The figure shows three views and two pictorial views of one solid part (mm, origin at its lowest corner). Answer the questions. Give positions to 0.01 mm unless a question says otherwise; leave off trailing zeros. Write each loop counter-clockwise with the first axis right and the second up, starting at its lowest first coordinate (ties: lowest second). Pieces come first, ordered by that corner, then holes. Notation, with made-up numbers: M 3.25,70.5 L 61.25,70.5 A15 cw 61.25,82.5 Z; hole C 34,81 d2. An arc over 180 degrees is marked long. Return JSON: item names as keys, results as strings.
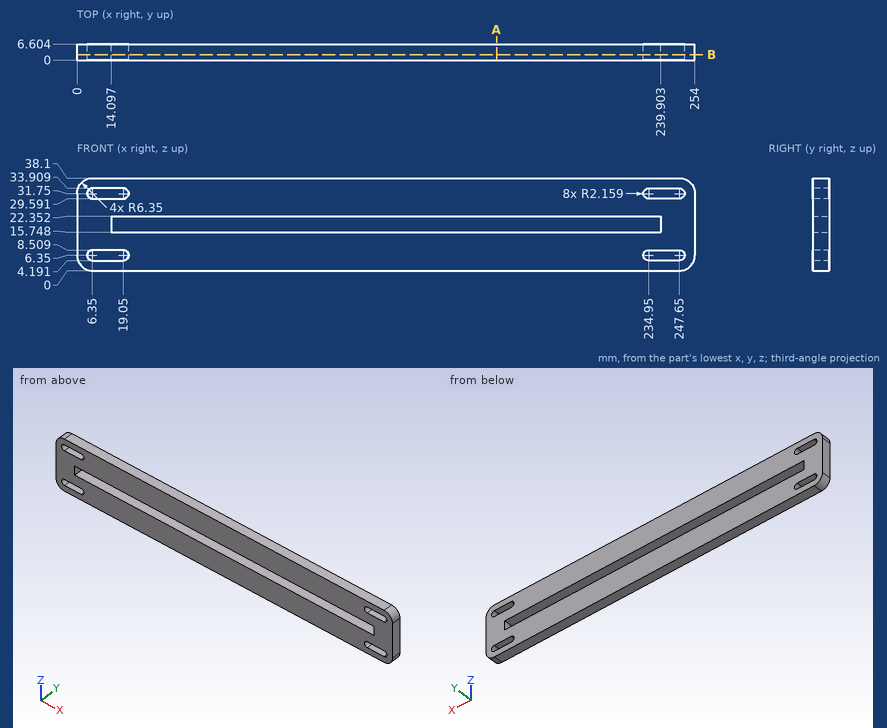
Item 1: A cutting plane is placed at B-B, the plane y = 2.25. Write down the section's boundary in (x, z).
Geometry results:
{"outline": "M 0,6.35 A6.35 ccw 6.35,0 L 247.65,0 A6.35 ccw 254,6.35 L 254,31.75 A6.35 ccw 247.65,38.1 L 6.35,38.1 A6.35 ccw 0,31.75 Z; hole M 6.35,4.19 L 19.05,4.19 A2.16 ccw 19.05,8.51 L 6.35,8.51 A2.16 ccw Z; hole M 6.35,29.59 L 19.05,29.59 A2.16 ccw 19.05,33.91 L 6.35,33.91 A2.16 ccw Z; hole M 14.1,15.75 L 239.9,15.75 L 239.9,22.35 L 14.1,22.35 Z; hole M 234.95,4.19 L 247.65,4.19 A2.16 ccw 247.65,8.51 L 234.95,8.51 A2.16 ccw Z; hole M 234.95,29.59 L 247.65,29.59 A2.16 ccw 247.65,33.91 L 234.95,33.91 A2.16 ccw Z"}
Item 2: Find the intervals of material crossed by line 1 (Z direction, x = 17.5, y = 3.25); line 2 (X direction, y = 4.5, z = 17.5); line 3 (Z direction, x = 67.5, y = 3.75), in increasing order.
Geometry results:
{"line 1": "z = 0 to 4.19, 8.51 to 15.75, 22.35 to 29.59, 33.91 to 38.1", "line 2": "x = 0 to 14.1, 239.9 to 254", "line 3": "z = 0 to 15.75, 22.35 to 38.1"}
Item 3: A cutting plane is placed at A-A, the plane x = 172.5. Write down the section's boundary in (y, z).
Geometry results:
{"outline": "M 0,0 L 6.6,0 L 6.6,15.75 L 0,15.75 Z; M 0,22.35 L 6.6,22.35 L 6.6,38.1 L 0,38.1 Z"}
